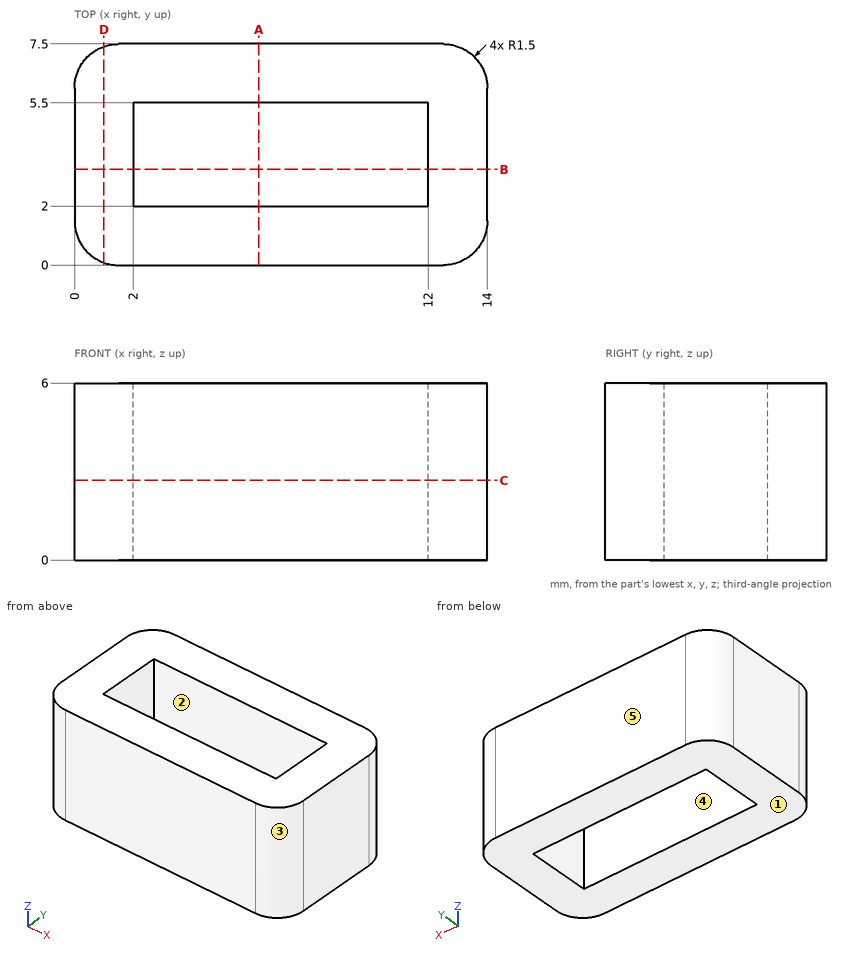
Here's the drawing with two shaded views (mm, measured from the low corner). I have some questions. A direction names the side the tool comes from. Give positions to 0.01 mm unless a question says otherwise; leave off trailing zeros. Loops run counter-clockwise (first coordinate to the right, second up) from the corner with the lowest first, then second, coordinate; pieces in that order, holes last. Notation, with made-up numbers: M -37.75,54 L -15.75,54 A7 cw -15.75,61 Z; hole C 2.5,28.5 d5. An arc over 180 degrees is marked long. One line per item, written item: value. Start each with the question number.
1) If we section it at D-D, the plane x = 1: Write out the boundary of the cut face in (y, z), and give its area (3 significant figures).
2) If I drill on line 1 (Y direction, x = 7.25, z = 4.85); line 2 (X direction, y = 3.5, z = 0.7); line 3 (X direction, y = 7, z = 5.75), over which ranges is the centre line in solid material (lowest first)? Write a range as [from, to].
3) If we section it at C-C, the plane z = 2.7: Write out the boundary of the cut face in (x, y).
4) On a 3-axis mill with a long thin cutter (end or side, diameter ignored), from which of +Z, -Z, +X, -X, +Y, -Y can I reach the whole of each face in a straight line? I mean the marked faces 4 and 5. Say none if no direction works.
5) Thinking about a two-plate mould opening in X: for the marked faces 1, 2 and 3, which applies, +X half, -X half, draft (parallel to the pull), parting line (faces both ways), or undercut?
6) If we section it at B-B, the plane y = 3.25: Write out the boundary of the cut face in (x, z), and give its area (3 significant figures).
7) If we section it at A-A, the plane x = 6.25: Write out the boundary of the cut face in (y, z), and give its area (3 significant figures).
Completed:
1. outline: M 0.09,0 L 7.41,0 L 7.41,6 L 0.09,6 Z
1. area: 44.0 mm^2
2. line 1: y = [0, 2], [5.5, 7.5]
2. line 2: x = [0, 2], [12, 14]
2. line 3: x = [0.38, 13.62]
3. outline: M 0,1.5 A1.5 ccw 1.5,0 L 12.5,0 A1.5 ccw 14,1.5 L 14,6 A1.5 ccw 12.5,7.5 L 1.5,7.5 A1.5 ccw 0,6 Z; hole M 2,2 L 12,2 L 12,5.5 L 2,5.5 Z
4. face 4: +Z, -Z
4. face 5: +Z, -Z, +X, -X, +Y
5. face 1: draft
5. face 2: undercut
5. face 3: +X half
6. outline: M 0,0 L 2,0 L 2,6 L 0,6 Z; M 12,0 L 14,0 L 14,6 L 12,6 Z
6. area: 24.0 mm^2
7. outline: M 0,0 L 2,0 L 2,6 L 0,6 Z; M 5.5,0 L 7.5,0 L 7.5,6 L 5.5,6 Z
7. area: 24.0 mm^2
